Work out the finished part from the listing and answer in its coordinate system (mm). A direction names the side the tool comes from. Give positions to 0.01 mm unless a question says otherwise; leave off trailing zeros. Order: outer loops, then holes, each group sorted by start corner. A loop starts at its lowest first (then second) coordinate and runs counter-clockwise, first axis right, second up. Notation, with made-up numbers: (48.25, 76.25) - (60.25, 76.25) arc R7 cw to (60.25, 87.25) - close; hole circle Ø6 at (-29, -36.75). An arc over 180 degrees is marked (long way). Return JSON: item names as keys, results as strings. Group by question number.
from build123d import *

# Parameters (mm, degrees)
SKETCH1_W          = 257.175
SKETCH1_H          = 76.2
SKETCH1_R          = 12.7
EXTRUDE1_DEPTH     = 12.7
CUT_EXTRUDE2_REACH = 142.572


with BuildPart() as part:
    # Sketch1 → Extrude1 (new, symmetric)
    with BuildSketch(Plane(origin=(0, 0, 0), x_dir=(0, 0, -1), z_dir=(1, 0, 0))):
        with Locations((0, 12.7)):
            Rectangle(SKETCH1_W, SKETCH1_H)
        with Locations((-103.1875, 0)):
            Circle(SKETCH1_R, mode=Mode.SUBTRACT)
        with Locations((103.1875, 0)):
            Circle(SKETCH1_R, mode=Mode.SUBTRACT)
    extrude(amount=EXTRUDE1_DEPTH, both=True)

    # Sketch2 → Cut-Extrude2 (cut, up to next)
    with BuildSketch(Plane(origin=(12.7, 0, 0), x_dir=(0, 0, -1), z_dir=(1, 0, 0)), mode=Mode.PRIVATE) as cut_extrude2_sk1:
        Polygon((-90.4875, -25.4), (-65.0875, 0), (65.0875, 0), (90.4875, -25.4), align=None)
    cut_extrude2_tool1 = extrude(cut_extrude2_sk1.sketch, amount=-CUT_EXTRUDE2_REACH, mode=Mode.PRIVATE) & part.part
    # Sketch2 → Cut-Extrude2 (cut, up to next)
    with BuildSketch(Plane(origin=(12.7, 0, 0), x_dir=(0, 0, -1), z_dir=(1, 0, 0)), mode=Mode.PRIVATE) as cut_extrude2_sk2:
        Polygon((-128.5875, 50.8), (-128.5875, 12.7), (-77.7875, 50.8), align=None)
    cut_extrude2_tool2 = extrude(cut_extrude2_sk2.sketch, amount=-CUT_EXTRUDE2_REACH, mode=Mode.PRIVATE) & part.part
    # Sketch2 → Cut-Extrude2 (cut, up to next)
    with BuildSketch(Plane(origin=(12.7, 0, 0), x_dir=(0, 0, -1), z_dir=(1, 0, 0)), mode=Mode.PRIVATE) as cut_extrude2_sk3:
        Polygon((77.7875, 50.8), (128.5875, 50.8), (128.5875, 12.7), align=None)
    cut_extrude2_tool3 = extrude(cut_extrude2_sk3.sketch, amount=-CUT_EXTRUDE2_REACH, mode=Mode.PRIVATE) & part.part
    # Sketch2 → Cut-Extrude2 (cut, up to next)
    with BuildSketch(Plane(origin=(12.7, 0, 0), x_dir=(0, 0, -1), z_dir=(1, 0, 0)), mode=Mode.PRIVATE) as cut_extrude2_sk4:
        Polygon((-128.5875, -25.4), (-128.5875, -12.7), (-115.8875, -25.4), align=None)
    cut_extrude2_tool4 = extrude(cut_extrude2_sk4.sketch, amount=-CUT_EXTRUDE2_REACH, mode=Mode.PRIVATE) & part.part
    # Sketch2 → Cut-Extrude2 (cut, up to next)
    with BuildSketch(Plane(origin=(12.7, 0, 0), x_dir=(0, 0, -1), z_dir=(1, 0, 0)), mode=Mode.PRIVATE) as cut_extrude2_sk5:
        Polygon((128.5875, -12.7), (128.5875, -25.4), (115.8875, -25.4), align=None)
    cut_extrude2_tool5 = extrude(cut_extrude2_sk5.sketch, amount=-CUT_EXTRUDE2_REACH, mode=Mode.PRIVATE) & part.part
    add(cut_extrude2_tool1.solids().sort_by_distance((12.7, -13.391156, 0))[0], mode=Mode.SUBTRACT)
    add(cut_extrude2_tool2.solids().sort_by_distance((12.7, 38.1, 111.654167))[0], mode=Mode.SUBTRACT)
    add(cut_extrude2_tool3.solids().sort_by_distance((12.7, 38.1, -111.654167))[0], mode=Mode.SUBTRACT)
    add(cut_extrude2_tool4.solids().sort_by_distance((12.7, -21.166667, 124.354167))[0], mode=Mode.SUBTRACT)
    add(cut_extrude2_tool5.solids().sort_by_distance((12.7, -21.166667, -124.354167))[0], mode=Mode.SUBTRACT)


solid = part.part
1. Each of these flat-tipped pins is pushed along its axis until it touches: pin 1 (1 mm diameter, centred on x = -5.5, z = -83, fed in from -Y); pin 2 (23 mm diameter, centred on y = 0, z = -103.19, fed in from +X); pin 3 (5 mm diameter, centred on x = -8.5, y = 42.5, fed in from -Z); pin 4 (1 mm diameter, centred on x = -9, y = -16, fed in from -Z). Where does it stop, or does it pass through?
2. Determine the mould class of faces 3 (the flat face through (12.7, 13, 2)), 4 (the flat face through (0.18, -18.96, 122.33)), 5 (the cylindrical face through (-0.178, 0.558, 115.875)), 6 (the cylindrical face through (-0.2, 0.6, -90.5)) for opening direction Y: released by +Y, released by -Y, zero draft, split by the parting line, or undercut.
3. A tool of negligible diameter and unlimited length cuts with its end or side. For faces 1 (the flat face through (0, -25.4, -103)), 2 (the flat face through (0, 0, 1)), from which of +Z, -Z, +X, -X, +Y, -Y can it reach the whole face along a straight path? Write none if from no direction.
4. The part is cut by section A-A (y = -17.5). Give the vertices of the cut face in (x, z), and give its area (3 significant figures).
5. The part is cut by section D-D (y = -8). Give the vertices of the cut face in (x, z), and give its area (3 significant figures).
6. The part is cut by section C-C (y = 9). Give the vertices of the cut face in (x, z), and give its area (3 significant figures).
7. Consider probe 1 along Y at (x, z) = (-2, -10); probe 2 along Z at (x, y) = (2, 3); probe 3 along Z at (x, y) = (-7.5, 2.5). Determine where each line is inside the solid, lowest interval first. Write a range as from..to.
8. The part is cut by section B-B (x = -2.5). Give the vertices of the cut face in (y, z).
Answers:
{
 "1": {"pin 1": "stops at y = -18.41", "pin 2": "passes through", "pin 3": "stops at z = -92.19", "pin 4": "stops at z = -125.79"},
 "2": {"face 3": "zero draft", "face 4": "released by -Y", "face 5": "undercut", "face 6": "undercut"},
 "3": {"face 1": "+Z, -Z, +X, -X, -Y", "face 2": "+X, -X, -Y"},
 "4": {"outline": "(-12.7, -123.79) - (12.7, -123.79) - (12.7, -82.59) - (-12.7, -82.59) - close; (-12.7, 82.59) - (12.7, 82.59) - (12.7, 123.79) - (-12.7, 123.79) - close", "area": "2,090 mm^2"},
 "5": {"outline": "(-12.7, -128.59) - (12.7, -128.59) - (12.7, -113.05) - (-12.7, -113.05) - close; (-12.7, -93.32) - (12.7, -93.32) - (12.7, -73.09) - (-12.7, -73.09) - close; (-12.7, 73.09) - (12.7, 73.09) - (12.7, 93.32) - (-12.7, 93.32) - close; (-12.7, 113.05) - (12.7, 113.05) - (12.7, 128.59) - (-12.7, 128.59) - close", "area": "1,820 mm^2"},
 "6": {"outline": "(-12.7, -128.59) - (12.7, -128.59) - (12.7, -112.15) - (-12.7, -112.15) - close; (-12.7, -94.23) - (12.7, -94.23) - (12.7, 94.23) - (-12.7, 94.23) - close; (-12.7, 112.15) - (12.7, 112.15) - (12.7, 128.59) - (-12.7, 128.59) - close", "area": "5,620 mm^2"},
 "7": {"probe 1": "y = 0..50.8", "probe 2": "z = -128.59..-115.53, -90.85..90.85, 115.53..128.59", "probe 3": "z = -128.59..-115.64, -90.74..90.74, 115.64..128.59"},
 "8": {"outline": "(-25.4, -115.89) - (-12.7, -128.59) - (12.7, -128.59) - (50.8, -77.79) - (50.8, 77.79) - (12.7, 128.59) - (-12.7, 128.59) - (-25.4, 115.89) - (-25.4, 90.49) - (0, 65.09) - (0, -65.09) - (-25.4, -90.49) - close; hole circle Ø25.4 at (0, -103.19); hole circle Ø25.4 at (0, 103.19)"}
}
